Work out the finished part from the listing and answer in its coordinate system (mm). A direction names the side the tool comes from. Round coordinates to 2 decimals unless told otherwise and drop trailing zeros. Loops run counter-clockwise (first coordinate to the right, second up) from the corner with the lowest first, then second, coordinate; pieces in that order, holes last. Notation, with made-up numbers: (40, -18.75) -> (82, -18.75) arc R21 ccw to (82, 20.25) -> close; hole circle Ø10 at (-38.75, -25.75). An arc over 180 degrees is marked (long way). Write item = value, one per line. Start each with the question number.
```python
from build123d import *

# Parameters (mm, degrees)
F1_DEPTH = 5
F3_D     = 4.4958
F4_R     = 2


with BuildPart() as f1:
    # F0 (on Top) → F1 (new body, symmetric)
    with BuildSketch(Plane.XY):
        with BuildLine():
            Line((0, 2.4), (0, 0))
            Line((0, 0), (47.5, 0))
            ThreePointArc((47.5, 0), (59.8036579926, 5.0963420074), (64.9, 17.4))
            Line((64.9, 17.4), (64.9, 34))
            Line((64.9, 34), (74.9, 34))
            Line((74.9, 34), (74.9, 36.4))
            Line((74.9, 36.4), (62.5, 36.4))
            Line((62.5, 36.4), (62.5, 17.4))
            ThreePointArc((62.5, 17.4), (58.1066017178, 6.7933982822), (47.5, 2.4))
            Line((47.5, 2.4), (0, 2.4))
        make_face()
    extrude(amount=F1_DEPTH, both=True)

    # F3 (through all)
    with Locations(Plane.XZ.offset(-34)):
        with Locations((69.9, 0)):
            Hole(F3_D / 2)

    # F4
    f4_edges = [f1.edges().sort_by_distance(p)[0] for p in [
        (64.9, 34, 0),
        (74.9, 34, 0),
    ]]
    fillet(f4_edges, radius=F4_R)

    # F5: F1 across face


with BuildPart() as f1_1:
    add(f1.part)
    add(f1.part.mirror(Plane(origin=(0, 1.2, 0), x_dir=(0, -1, 0), z_dir=(-1, 0, 0))))


solid = f1_1.part
```
Item 1: Find the intervals of material crossed by line 1 along Z through (x, y) = (-69.9, 34.5); line 2 along X through (y, z) = (20.5, 2.75); line 3 along Y through (x, z) = (17, -1), in increasing order. Write a range as [from, to].
Item 2: A tool of negligible diameter and unlimited length cuts with its end or side. For faces 1 (the flat face through (-64.9, 25, 0)), 2 (the flat face through (62.5, 27, 0)), 3 (the flat face through (64.9, 25, 0)), 4 (the cylindrical face through (67.756, 35.217, 0.675)), from which of +Z, -Z, +X, -X, +Y, -Y can it reach the whole face along a straight path? Write none if from no direction.
Item 3: The mould has two halves that part along X. Classify faces 5 (the flat face through (-62.5, 27, 0)), 6 (the flat face through (1, 0, 0)), 7 (the cylindrical face through (59.668, 4.962, 0.07)): pulls with the +X half, pulls with the -X half, needs draft (parallel to the pull), parting line crosses it, or undercut.
Item 4: Section A-A (z = 0) is taken. Determine the outline of the cut face in (x, y), then the cut area to 3 significant figures.
Item 5: Section D-D (x = 36.5) is taken. Determine the outline of the cut face in (y, z), then the cut area to 3 significant figures.
Item 6: Section B-B (y = 19) is taken. Determine the outline of the cut face in (x, z).
Item 7: Section C-C (x = -69.9) is taken. Determine the outline of the cut face in (y, z).
Item 8: Flat-ended cylindrical pins translate along their axes: pin 1 (5 mm diameter, centred on x = -69, z = -0.5, fed in from -Y); pin 2 (4 mm diameter, centred on y = 25.5, z = -2, fed in from +X); pin 3 (10 mm diameter, centred on x = 53, y = 6.5, fed in from +Z); pin 4 (1 mm diameter, centred on y = 7, z = 3.5, fed in from +X). Find the tip coordinate at first contact, or state that the pin passes through.
Worked answers:
q1.line_1 = [-5, -2.25], [2.25, 5]
q1.line_2 = [-64.9, -62.5], [62.5, 64.9]
q1.line_3 = [0, 2.4]
q2.face_1 = +Z, -Z, -X, -Y
q2.face_2 = +Z, -Z, +Y
q2.face_3 = +Z, -Z, +X, -Y
q2.face_4 = +Y, -Y
q3.face_5 = undercut
q3.face_6 = needs draft
q3.face_7 = pulls with the +X half
q4.outline = (-74.9, 36) arc R2 ccw to (-72.9, 34) -> (-72.15, 34) -> (-72.15, 36.4) -> (-74.9, 36.4) -> close; (-67.65, 34) -> (-66.9, 34) arc R2 cw to (-64.9, 32) -> (-64.9, 17.4) arc R17.4 ccw to (-47.5, 0) -> (47.5, 0) arc R17.4 ccw to (64.9, 17.4) -> (64.9, 32) arc R2 cw to (66.9, 34) -> (67.65, 34) -> (67.65, 36.4) -> (62.5, 36.4) -> (62.5, 17.4) arc R15 cw to (47.5, 2.4) -> (-47.5, 2.4) arc R15 cw to (-62.5, 17.4) -> (-62.5, 36.4) -> (-67.65, 36.4) -> close; (72.15, 34) -> (72.9, 34) arc R2 ccw to (74.9, 36) -> (74.9, 36.4) -> (72.15, 36.4) -> close
q4.area = 468 mm2
q5.outline = (0, -5) -> (2.4, -5) -> (2.4, 5) -> (0, 5) -> close
q5.area = 24.0 mm2
q6.outline = (-64.9, -5) -> (-62.5, -5) -> (-62.5, 5) -> (-64.9, 5) -> close; (62.5, -5) -> (64.9, -5) -> (64.9, 5) -> (62.5, 5) -> close
q7.outline = (34, -5) -> (36.4, -5) -> (36.4, -2.25) -> (34, -2.25) -> close; (34, 2.25) -> (36.4, 2.25) -> (36.4, 5) -> (34, 5) -> close
q8.pin_1 = 33.96
q8.pin_2 = 64.9
q8.pin_3 = 5
q8.pin_4 = 61.81
